The model under review builds one solid part; all positions refer to its coordinate system, in mm. Face numbers are marked on the shaded views. A direction names the side the tool comes from. Round coordinates to 2 decimals unless told otherwise and drop trailing zeros. Order: outer loops, then holes, each group sorted by start corner. A loop starts at its lowest first (then second) coordinate and runs counter-clockwise, first axis right, second up. Notation, with made-up numbers: M 34,74.25 L 92,74.25 A24 cw 92,108.25 Z; hole C -22,65.5 d10. An arc over 180 degrees is marked long. Use a Markdown table: item, result. Add a question column.
1. Insertion check: P1, Ø2, axis at x = -4.5, y = 21, coming from the -Z side; P2, Ø5, axis at x = 25.5, z = 26, coming from the -Y side; P3, Ø6.5, axis at x = 23, y = 27, coming from the -Z side; P4, Ø1.5, axis at y = 14.5, z = 1.5, coming from the -X side. Each pin has a flat end and moves straight along its axis. Give the tip position at first contact, or say it passes through.
2. The part is to be moulded in two halves that separate along X. For the marked faces 1, 2 and 3, say which applies: +X half, -X half, draft (parallel to the pull), parting line (faces both ways), or undercut.
3. Consider section D-D on z = 27. Count the separate pieces of the cut face and the enclosed holes in it, then the cut area to 3 significant figures.
4. Consider section A-A on z = 40.5. State the section outline as (x, y) points.
5. Consider section C-C on y = 7. State the section outline as (x, z) points.
6. For the marked faces 4, 5, 6, 7 and 8, list the 3-axis set-ups (+Z, -Z, +X, -X, +Y, -Y) from which the entire face can be reached by the end or side of a thin tool; tool diameter is ignored.
7. To check wall thickness, follow probe 1 along Z at (x, y) = (-38, 7); probe 2 along X at (y, z) = (-4, 18.5); probe 3 along Z at (x, y) = (28.5, 11). State the ranges of each line that lie inside material, in increasing order.
8. Consider section B-B on x = 26. State the section outline as (y, z) points, then the cut area to 3 significant figures.
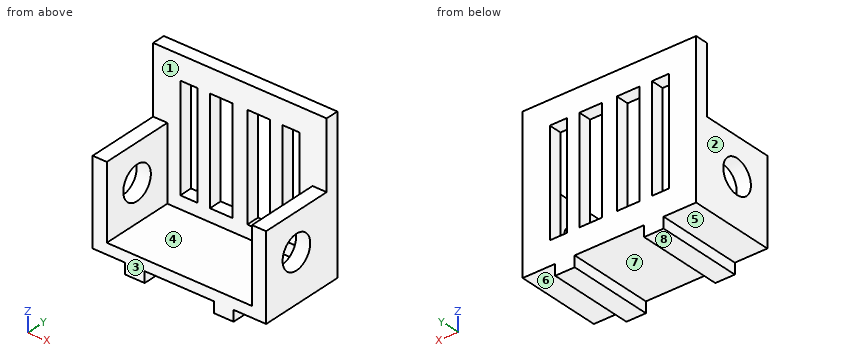
from build123d import *

# Parameters (mm, degrees)
F0_W      = 80
F0_H      = 60
F1_DEPTH  = 10
F2_W      = 15
F2_H      = 60
F2_W_2    = 32
F3_DEPTH  = 5
F4_W      = 80
F4_H      = 6
F5_DEPTH  = 65
F7_W      = 7.8638531268
F7_H      = 48.2417996228
F7_W_2    = 10.3811963927
F8_DEPTH  = 25
F9_W      = 6.5171729342
F9_H      = 34
F10_DEPTH = 34
F11_R     = 7.75
F13_DEPTH = 25
F14_W     = 20
F14_H     = 5
F15_DEPTH = 90
F16_W     = 20
F16_H     = 5
F17_DEPTH = 25
F18_W     = 20
F18_H     = 5
F19_DEPTH = 25
F12_R     = 7.75
F20_DEPTH = 25


with BuildPart() as f1:
    # F0 (on Top) → F1 (new body)
    with BuildSketch(Plane.XY):
        Rectangle(F0_W, F0_H)
    extrude(amount=F1_DEPTH)

    # F2 (on face) → F3 (cut)
    with BuildSketch(Plane(origin=(0, 0, 0), x_dir=(1, 0, 0), z_dir=(0, 0, -1))):
        with Locations((32.5, 0)):
            Rectangle(F2_W, F2_H)
        Rectangle(F2_W_2, F2_H)
        with Locations((-32.5, 0)):
            Rectangle(F2_W, F2_H)
    extrude(amount=-F3_DEPTH, mode=Mode.SUBTRACT)

    # F4 (on face) → F5 (join)
    with BuildSketch(Plane.XY.offset(10)):
        with Locations((0, 27)):
            Rectangle(F4_W, F4_H)
    extrude(amount=F5_DEPTH)

    # F7 (on face) → F8 (cut)
    with BuildSketch(Plane(origin=(0, 30, 0), x_dir=(-1, 0, 0), z_dir=(0, 1, 0))):
        with Locations((-23.5581696033, 40)):
            Rectangle(F7_W, F7_H)
        with Locations((-8.6212871829, 40)):
            Rectangle(F7_W_2, F7_H)
        with Locations((8.6212871829, 40)):
            Rectangle(F7_W_2, F7_H)
        with Locations((23.5581696033, 40)):
            Rectangle(F7_W, F7_H)
    extrude(amount=-F8_DEPTH, mode=Mode.SUBTRACT)

    # F9 (on face) → F10 (join)
    with BuildSketch(Plane.XY.offset(10)):
        with Locations((-36.7414135329, 7)):
            Rectangle(F9_W, F9_H)
        with Locations((36.7414135329, 7)):
            Rectangle(F9_W, F9_H)
    extrude(amount=F10_DEPTH)

    # F11 (on face) → F13 (cut)
    with BuildSketch(Plane(origin=(-40, 0, 0), x_dir=(0, -1, 0), z_dir=(-1, 0, 0))):
        with Locations((-7, 27)):
            Circle(F11_R)
    extrude(amount=-F13_DEPTH, mode=Mode.SUBTRACT)

    # F14 (on face) → F15 (cut)
    with BuildSketch(Plane.YZ.offset(40)):
        with Locations((-20, 7.5)):
            Rectangle(F14_W, F14_H)
    extrude(amount=-F15_DEPTH, mode=Mode.SUBTRACT)

    # F16 (on face) → F17 (cut)
    with BuildSketch(Plane.YZ.offset(25)):
        with Locations((-20, 2.5)):
            Rectangle(F16_W, F16_H)
    extrude(amount=-F17_DEPTH, mode=Mode.SUBTRACT)

    # F18 (on face) → F19 (cut)
    with BuildSketch(Plane(origin=(-25, 0, 0), x_dir=(0, -1, 0), z_dir=(-1, 0, 0))):
        with Locations((20, 2.5)):
            Rectangle(F18_W, F18_H)
    extrude(amount=-F19_DEPTH, mode=Mode.SUBTRACT)

    # F12 (on face) → F20 (cut)
    with BuildSketch(Plane.YZ.offset(40)):
        with Locations((7, 27)):
            Circle(F12_R)
    extrude(amount=-F20_DEPTH, mode=Mode.SUBTRACT)


solid = f1.part
Answer block:
| question | item | result |
|---|---|---|
| 1 | P1 | z = 5 |
| 1 | P2 | y = 24 |
| 1 | P3 | z = 0 |
| 1 | P4 | x = -25 |
| 2 | face 1 | undercut |
| 2 | face 2 | -X half |
| 2 | face 3 | draft |
| 3 | separate pieces | 7 |
| 3 | enclosed holes | 0 |
| 3 | area | 502 mm^2 |
| 4 | outline | M -40,-10 L -33.48,-10 L -33.48,24 L -27.49,24 L -27.49,30 L -40,30 Z; M -19.63,24 L -13.81,24 L -13.81,30 L -19.63,30 Z; M -3.43,24 L 3.43,24 L 3.43,30 L -3.43,30 Z; M 13.81,24 L 19.63,24 L 19.63,30 L 13.81,30 Z; M 27.49,24 L 33.48,24 L 33.48,-10 L 40,-10 L 40,30 L 27.49,30 Z |
| 5 | outline | M -40,5 L -25,5 L -25,0 L -16,0 L -16,5 L 16,5 L 16,0 L 25,0 L 25,5 L 40,5 L 40,19.25 L 33.48,19.25 L 33.48,10 L -33.48,10 L -33.48,19.25 L -40,19.25 Z; M -40,34.75 L -33.48,34.75 L -33.48,44 L -40,44 Z; M 33.48,34.75 L 40,34.75 L 40,44 L 33.48,44 Z |
| 6 | face 4 | +Z, -Y |
| 6 | face 5 | -Z, -X, +Y, -Y |
| 6 | face 6 | -Z, +X, +Y, -Y |
| 6 | face 7 | -Z, +Y, -Y |
| 6 | face 8 | -Z, +X, -X, +Y, -Y |
| 7 | probe 1 | 5 to 19.25, 34.75 to 44 |
| 7 | probe 2 | -40 to -33.48, 33.48 to 40 |
| 7 | probe 3 | 5 to 10 |
| 8 | outline | M -10,5 L 30,5 L 30,15.88 L 24,15.88 L 24,10 L -10,10 Z; M 24,64.12 L 30,64.12 L 30,75 L 24,75 Z |
| 8 | area | 301 mm^2 |
